Design review of the part built by this model. Coordinates are the model's own, in mm. A direction names the side the tool comes from. Coordinates: 2 decimals unless noted, no trailing zeros. Loops run counter-clockwise (first coordinate to the right, second up) from the corner with the lowest first, then second, coordinate; pieces in that order, holes last.
Q1. For P1, Ø8, axis at x = -22.5, y = -8, coming from the +Z side; P2, Ø10, axis at y = -51, z = 13, coming from the +X side; P3, Ø9, axis at x = 11.5, z = 14.5, coming from the -Y side (3 decimals), all flat-tipped, find the tip position at first contact; note any pin that passes through.
Q2. Add section C-C on y = 42.5. Give the boundary of the cut face in (x, z).
Q3. Add section B-B on x = -20.5. Give the boundary of the cut face in (y, z) (3 decimals), and give its area (3 significant figures).
Q4. Add section A-A on z = 23. Give the boundary of the cut face in (x, y) (3 decimals).
Q5. Draft analysis for pull direction X (two halves, no side actions). For faces 1 (the face through (50.036, -34.201, 18.637)), 2 (the face through (-1, 1, 0)), 3 (the face through (-47.496, 57.061, 19.481)), 4 (the face through (-3.264, -57.021, 19.481)), state which applies: released by +X, released by -X, zero draft, split by the parting line, or undercut.
Q6. Wall thickness on probe 1 along Y at (x, z) = (-42.5, 11) (3 decimals); probe 2 along X at (y, z) = (-38, 29.5); probe 3 along X at (y, z) = (-6.5, 27): over which ranges is each line inside the solid? List them lowest first.
Q7. Machinability: for faces 5 (the face through (50.8, 12, 18)), 6 (the face through (25.72, -34.161, 0.724)), 7 (the face through (-50.036, -0.809, 0.724)), 8 (the face through (0, -48, 18)), 9 (the face through (-1, 1, 2.54)), which of the approach directions +Z, -Z, +X, -X, +Y, -Y give a long, thin tool a straight path to every point of the face, cutting with its end or side? Answer none if there is none.
```python
from build123d import *

# Parameters (mm, degrees)
F1_DEPTH = 34.29
F3_DEPTH = 31.75
F4_W     = 10.16
F4_H     = 7.62
F5_DEPTH = 2.54
F6_R     = 0.127
F7_R     = 2.54


with BuildPart() as f1:
    # F0 (on Top) → F1 (new body)
    with BuildSketch(Plane.XY):
        Polygon((50.8, 60.325), (-50.8, 60.325), (-50.8, -60.325), (0, -60.325), (0, -34.925), (50.8, -34.925), align=None)
    extrude(amount=F1_DEPTH)

    # F2 (on face) → F3 (cut)
    with BuildSketch(Plane.XY.offset(34.29)):
        Polygon((48.26, -32.385), (48.26, 57.785), (-48.26, 57.785), (-48.26, -57.785), (-2.54, -57.785), (-2.54, -32.385), align=None)
    extrude(amount=-F3_DEPTH, mode=Mode.SUBTRACT)

    # F4 (on face) → F5 (cut, through all)
    with BuildSketch(Plane.YZ):
        with Locations((-45.085, 12.7)):
            Rectangle(F4_W, F4_H)
    extrude(amount=-F5_DEPTH, mode=Mode.SUBTRACT)

    # F6
    f6_edges = [f1.edges().sort_by_distance(p)[0] for p in [
        (-1.27, -50.165, 16.51),
        (-1.27, -40.005, 16.51),
        (-1.27, -40.005, 8.89),
        (-1.27, -50.165, 8.89),
    ]]
    fillet(f6_edges, radius=F6_R)

    # F7
    f7_edges = [f1.edges().sort_by_distance(p)[0] for p in [
        (50.8, -34.925, 17.145),
        (0, -34.925, 17.145),
        (0, -60.325, 17.145),
        (-2.54, -32.385, 18.415),
        (-50.8, -60.325, 17.145),
        (-2.54, -57.785, 18.415),
        (-48.26, -57.785, 18.415),
        (50.8, 60.325, 17.145),
        (48.26, 57.785, 18.415),
        (-48.26, 57.785, 18.415),
        (-50.8, 60.325, 17.145),
        (0, 60.325, 0),
        (-50.8, 0, 0),
        (-25.4, -60.325, 0),
        (0, -47.625, 0),
        (25.4, -34.925, 0),
        (50.8, 12.7, 0),
        (48.26, 12.7, 2.54),
        (0, 57.785, 2.54),
        (-48.26, 0, 2.54),
        (-25.4, -57.785, 2.54),
        (-2.54, -45.085, 2.54),
        (22.86, -32.385, 2.54),
    ]]
    fillet(f7_edges, radius=F7_R)


solid = f1.part
```
Entries:
1. P1: stops at z = 2.54
1. P2: stops at x = 0
1. P3: stops at y = -34.925
2. outline: (-50.8, 2.54) arc R2.54 ccw to (-48.26, 0) - (48.26, 0) arc R2.54 ccw to (50.8, 2.54) - (50.8, 34.29) - (48.26, 34.29) - (48.26, 5.08) arc R2.54 cw to (45.72, 2.54) - (-45.72, 2.54) arc R2.54 cw to (-48.26, 5.08) - (-48.26, 34.29) - (-50.8, 34.29) - close
3. outline: (-60.325, 2.54) arc R2.54 ccw to (-57.785, 0) - (57.785, 0) arc R2.54 ccw to (60.325, 2.54) - (60.325, 34.29) - (57.785, 34.29) - (57.785, 5.08) arc R2.54 cw to (55.245, 2.54) - (-55.245, 2.54) arc R2.54 cw to (-57.785, 5.08) - (-57.785, 34.29) - (-60.325, 34.29) - close
3. area: 468 mm2
4. outline: (-50.8, -57.785) arc R2.54 ccw to (-48.26, -60.325) - (-2.54, -60.325) arc R2.54 ccw to (0, -57.785) - (0, -37.465) arc R2.54 cw to (2.54, -34.925) - (48.26, -34.925) arc R2.54 ccw to (50.8, -32.385) - (50.8, 57.785) arc R2.54 ccw to (48.26, 60.325) - (-48.26, 60.325) arc R2.54 ccw to (-50.8, 57.785) - close; hole (-48.26, -55.245) arc R2.54 ccw to (-45.72, -57.785) - (-5.08, -57.785) arc R2.54 ccw to (-2.54, -55.245) - (-2.54, -34.925) arc R2.54 cw to (0, -32.385) - (48.26, -32.385) - (48.26, 55.245) arc R2.54 ccw to (45.72, 57.785) - (-45.72, 57.785) arc R2.54 ccw to (-48.26, 55.245) - close
5. face 1: released by +X
5. face 2: zero draft
5. face 3: undercut
5. face 4: undercut
6. probe 1: y = -60.325 to -57.785, 57.785 to 60.325
6. probe 2: x = -50.8 to -48.26, -2.54 to 0
6. probe 3: x = -50.8 to -48.26, 48.26 to 50.8
7. face 5: +Z, -Z, +X, +Y, -Y
7. face 6: -Z, +X, -Y
7. face 7: -Z, -X, +Y, -Y
7. face 8: +Z, -Z, +X, -Y
7. face 9: +Z
